Autodesk Inventor part; units mm, degrees
ref_plane "Plano de trabajo6" through (1679.9933, 1360, 0) normal (0, -1, 0) x (1, 0, 0)
ref_plane "YZ Plane" through (0, 0, 0) normal (1, 0, 0) x (0, 1, 0)
ref_plane "XZ Plane" through (0, 0, 0) normal (0, 1, 0) x (-1, 0, 0)
sketch "Boceto1" plane through (0, 0, 0) normal (0, 0, 1) x (1, 0, 0)
  line L0 (-332.0752, 0) -> (-331.8519, -0.5171)
  line L1 (560.0067, 1140) -> (559.9933, 1139.483)
  line L2 (332.0752, 0) -> (331.8519, -0.5171)
  line L3 (559.9933, 488.7901) -> (559.9933, 1360)
  line L4 (559.9933, 1360) -> (565.6963, 1360)
  line L5 (1679.9933, 1360) -> (1679.9933, 490)
  line L6 (1397.0917, 0) -> (842.9014, 0)
  line L7 (559.9933, 490) -> (559.9933, 1360)
  line L8 (-277.7918, 0) -> (-277.7902, -0.0027)
  line L9 (1679.9933, 1360) -> (1679.9933, 1303.9992)
  line L10 (1679.9933, 1360) -> (1679.9933, 490)
  line L11 (1679.9933, 490) -> (1397.0917, 0)
  line L12 (559.9933, 1360) -> (559.9933, 490)
  line L13 (559.9933, 490) -> (842.9014, 0)
  point P0 (0, 0)
  point P1 (0, -20)
  point P2 (277.7902, 0)
ref_plane "Plano de trabajo6" through (1679.9933, 1360, 0) normal (0, -1, 0) x (1, 0, 0)
sketch "Boceto7" plane through (1679.9933, 1360, 0) normal (0, -1, 0) x (1, 0, 0)
  circle A0 centre (0, 0) radius 21
  circle A1 centre (0, 0) radius 19.2
  point P0 (-1679.9933, 0)
  dimension "d32" = 42
  dimension "d33" = 38.4
sweep "Barrido3" add profiles "Boceto7" path "Boceto1" path curves L5 L11 L6 L13 L12
properties part number "barra_palanca" material "Acero, carbono"
Build history of the part. All positions in model axes, mm. A direction names the side the tool comes from. Round coordinates to 2 decimals unless told otherwise and drop trailing zeros. Write each loop counter-clockwise with the first axis right and the second up, starting at its lowest first coordinate (ties: lowest second). Pieces come first, ordered by that corner, then holes. Notation, with made-up numbers: M 9,-31.5 L 18,-31.5 A20 ccw 18,-25.5 Z; hole C 57,82 d6. An arc over 180 degrees is marked long. Answer as a JSON object with one key per item and string values. Group by question number.
(1) Cut at A-A (z = 0). Give the cut face in (x, y).
(2) Mould opens along X. For faces 1 (the flat face through (550.76, 1360, 17.01)), 2 (the cylindrical face through (717.507, 255.547, 0.844)) say: pulls with the +X half, pulls with the -X half, needs draft (parallel to the pull), parting line crosses it, or undercut.
(3) Which spindle directions (+Z, -Z, +X, -X, +Y, -Y) get a long thin tool onto all of the face, cutting with end or side? Do faces 3 (the cylindrical face through (1115.95, -20.03, 6.31)), 4 (the flat face through (1670.76, 1360, -17.01)), 5 (the cylindrical face through (1700.024, 916.057, 6.308)). Say none if no direction does.
(4) Flat gauge pins, fed straight in: pin 1 (3 mm diameter, centred on y = 1114, z = 12.5, fed in from +X); pin 2 (2 mm diameter, centred on x = 787.5, z = 14.5, fed in from -Y); pin 3 (12 mm diameter, centred on x = 915, z = 14.5, fed in from -Y). Where does each tip first touch, or does it go through?
(5) Drill centre lines: L1, parallel to X at y = 776.5, z = 2; L2, parallel to X at y = 757, z = 0; L3, parallel to Y at x = 1277, z = 0. Where is each one in solid material? Low to high.
(6) Cut at B-B (y = 244.5). Give the number of separate pieces and of enclosed holes in the cut face, and give its area (3 significant figures).
Responses:
{
 "1": {"outline": "M 538.99,484.37 L 830.78,-21 L 1409.22,-21 L 1700.99,484.37 L 1700.99,1360 L 1699.19,1360 L 1699.19,484.86 L 1408.18,-19.2 L 831.82,-19.2 L 540.79,484.86 L 540.79,1360 L 538.99,1360 Z; M 579.19,495.14 L 853.99,19.2 L 1386.01,19.2 L 1660.79,495.14 L 1660.79,1360 L 1658.99,1360 L 1658.99,495.63 L 1384.97,21 L 855.03,21 L 580.99,495.63 L 580.99,1360 L 579.19,1360 Z"},
 "2": {"face 1": "needs draft", "face 2": "undercut"},
 "3": {"face 3": "none", "face 4": "+Z, -Z, +X, -X, +Y", "face 5": "+Y"},
 "4": {"pin 1": "stops at x = 1697.88", "pin 2": "stops at y = 63.06", "pin 3": "stops at y = -19.2"},
 "5": {"L1": "x = 539.09 to 540.9, 579.09 to 580.9, 1659.09 to 1660.9, 1699.09 to 1700.9", "L2": "x = 538.99 to 540.79, 579.19 to 580.99, 1658.99 to 1660.79, 1699.19 to 1700.99", "L3": "y = -21 to -19.2, 19.2 to 21"},
 "6": {"separate pieces": "2", "enclosed holes": "2", "area": "525 mm2"}
}
